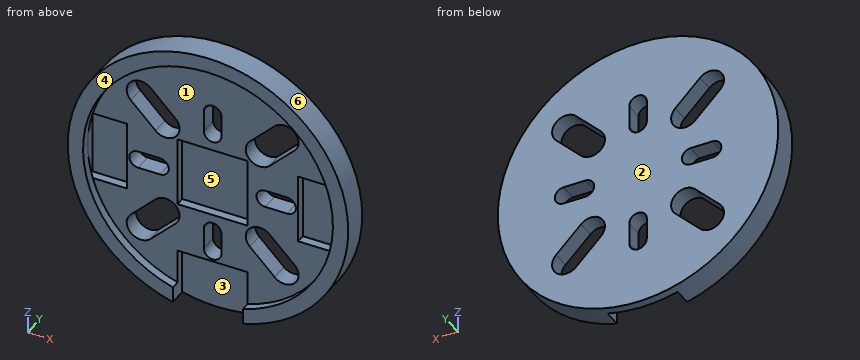
from build123d import *

# Parameters (mm, degrees)
F0_R     = 16
F1_DEPTH = 3
F3_DEPTH = 1
F4_W     = 8
F4_H     = 8
F4_W_2   = 4.5
F5_DEPTH = 1
F7_DEPTH = 3.001
F9_DEPTH = 3.001


with BuildPart() as f1:
    # F0 (on Front) → F1 (new body)
    with BuildSketch(Plane.XZ):
        Circle(F0_R)
    extrude(amount=F1_DEPTH)

    # F2 (on face) → F3 (cut)
    with BuildSketch(Plane.XZ.offset(3)):
        with BuildLine():
            Line((4, -16.6770793666), (4, -13.6770793666))
            ThreePointArc((4, -13.6770793666), (0, 14.25), (-4, -13.6770793666))
            Line((-4, -13.6770793666), (-4, -16.6770793666))
            Line((-4, -16.6770793666), (4, -16.6770793666))
        make_face()
    extrude(amount=-F3_DEPTH, mode=Mode.SUBTRACT)

    # F4 (on face) → F5 (cut)
    with BuildSketch(Plane.XZ.offset(2)):
        Rectangle(F4_W, F4_H)
        with Locations((-12, 0)):
            Rectangle(F4_W_2, F4_H)
        with Locations((12, 0)):
            Rectangle(F4_W_2, F4_H)
        with BuildLine():
            Line((4, -13.6770793666), (4, -9.75))
            Line((4, -9.75), (-4, -9.75))
            Line((-4, -9.75), (-4, -13.6770793666))
            Line((-4, -13.6770793666), (-4, -14.25))
            Line((-4, -14.25), (-4, -15.4919333848))
            ThreePointArc((-4, -15.4919333848), (0, -16), (4, -15.4919333848))
            Line((4, -15.4919333848), (4, -14.25))
            Line((4, -14.25), (4, -13.6770793666))
        make_face()
    extrude(amount=-F5_DEPTH, mode=Mode.SUBTRACT)

    # F6 (on face) → F7 (cut, through all)
    with BuildSketch(Plane(origin=(0, 0, 0), x_dir=(-1, 0, 0), z_dir=(0, 1, 0))):
        with BuildLine():
            Line((1, 6), (1, 8.5))
            ThreePointArc((1, 8.5), (0, 9.5), (-1, 8.5))
            Line((-1, 8.5), (-1, 6))
            ThreePointArc((-1, 6), (0, 5), (1, 6))
        make_face()
        with BuildLine():
            ThreePointArc((-8.5, 1), (-9.5, 0), (-8.5, -1))
            Line((-8.5, -1), (-6, -1))
            ThreePointArc((-6, -1), (-5, 0), (-6, 1))
            Line((-6, 1), (-8.5, 1))
        make_face()
        with BuildLine():
            ThreePointArc((-1, -8.5), (0, -9.5), (1, -8.5))
            Line((1, -8.5), (1, -6))
            ThreePointArc((1, -6), (0, -5), (-1, -6))
            Line((-1, -6), (-1, -8.5))
        make_face()
        with BuildLine():
            ThreePointArc((8.5, -1), (9.5, 0), (8.5, 1))
            Line((8.5, 1), (6, 1))
            ThreePointArc((6, 1), (5, 0), (6, -1))
            Line((6, -1), (8.5, -1))
        make_face()
    extrude(amount=-F7_DEPTH, mode=Mode.SUBTRACT)

    # F8 (on face) → F9 (cut, through all)
    with BuildSketch(Plane(origin=(0, 0, 0), x_dir=(-1, 0, 0), z_dir=(0, 1, 0))):
        with BuildLine():
            ThreePointArc((-7.0710678119, -9.3338095117), (-6.7242314097, -8.8147321535), (-6.6024386618, -8.2024386618))
            ThreePointArc((-6.6024386618, -8.2024386618), (-7.59014517, -6.7242314097), (-9.3338095117, -7.0710678119))
            ThreePointArc((-9.3338095117, -7.0710678119), (-9.3338095117, -9.3338095117), (-7.0710678119, -9.3338095117))
        make_face()
        with BuildLine():
            ThreePointArc((-9.3338095117, -7.0710678119), (-7.59014517, -6.7242314097), (-6.6024386618, -8.2024386618))
            ThreePointArc((-6.6024386618, -8.2024386618), (-6.7242314097, -8.8147321535), (-7.0710678119, -9.3338095117))
            Line((-7.0710678119, -9.3338095117), (-4.2426406871, -6.5053823869))
            ThreePointArc((-4.2426406871, -6.5053823869), (-6.5053823869, -6.5053823869), (-6.5053823869, -4.2426406871))
            Line((-6.5053823869, -4.2426406871), (-9.3338095117, -7.0710678119))
        make_face()
        with BuildLine():
            ThreePointArc((-3.774011537, -5.374011537), (-4.7617180452, -3.895804285), (-6.5053823869, -4.2426406871))
            ThreePointArc((-6.5053823869, -4.2426406871), (-6.5053823869, -6.5053823869), (-4.2426406871, -6.5053823869))
            ThreePointArc((-4.2426406871, -6.5053823869), (-3.895804285, -5.9863050288), (-3.774011537, -5.374011537))
        make_face()
        with BuildLine():
            Line((9.3338095117, -7.0710678119), (6.5053823869, -4.2426406871))
            ThreePointArc((6.5053823869, -4.2426406871), (6.852218789, -4.7617180452), (6.974011537, -5.374011537))
            ThreePointArc((6.974011537, -5.374011537), (5.9863050288, -6.852218789), (4.2426406871, -6.5053823869))
            Line((4.2426406871, -6.5053823869), (7.0710678119, -9.3338095117))
            ThreePointArc((7.0710678119, -9.3338095117), (7.0710678119, -7.0710678119), (9.3338095117, -7.0710678119))
        make_face()
        with BuildLine():
            ThreePointArc((6.974011537, -5.374011537), (6.852218789, -4.7617180452), (6.5053823869, -4.2426406871))
            ThreePointArc((6.5053823869, -4.2426406871), (4.2426406871, -4.2426406871), (4.2426406871, -6.5053823869))
            ThreePointArc((4.2426406871, -6.5053823869), (5.9863050288, -6.852218789), (6.974011537, -5.374011537))
        make_face()
        with BuildLine():
            ThreePointArc((9.8024386618, -8.2024386618), (9.6806459138, -7.59014517), (9.3338095117, -7.0710678119))
            ThreePointArc((9.3338095117, -7.0710678119), (7.0710678119, -7.0710678119), (7.0710678119, -9.3338095117))
            ThreePointArc((7.0710678119, -9.3338095117), (8.8147321535, -9.6806459138), (9.8024386618, -8.2024386618))
        make_face()
        with BuildLine():
            Line((7.0710678119, 9.3338095117), (4.2426406871, 6.5053823869))
            ThreePointArc((4.2426406871, 6.5053823869), (5.9863050288, 6.852218789), (6.974011537, 5.374011537))
            ThreePointArc((6.974011537, 5.374011537), (6.852218789, 4.7617180452), (6.5053823869, 4.2426406871))
            Line((6.5053823869, 4.2426406871), (9.3338095117, 7.0710678119))
            ThreePointArc((9.3338095117, 7.0710678119), (7.0710678119, 7.0710678119), (7.0710678119, 9.3338095117))
        make_face()
        with BuildLine():
            ThreePointArc((6.974011537, 5.374011537), (5.9863050288, 6.852218789), (4.2426406871, 6.5053823869))
            ThreePointArc((4.2426406871, 6.5053823869), (4.2426406871, 4.2426406871), (6.5053823869, 4.2426406871))
            ThreePointArc((6.5053823869, 4.2426406871), (6.852218789, 4.7617180452), (6.974011537, 5.374011537))
        make_face()
        with BuildLine():
            ThreePointArc((9.8024386618, 8.2024386618), (8.8147321535, 9.6806459138), (7.0710678119, 9.3338095117))
            ThreePointArc((7.0710678119, 9.3338095117), (7.0710678119, 7.0710678119), (9.3338095117, 7.0710678119))
            ThreePointArc((9.3338095117, 7.0710678119), (9.6806459138, 7.59014517), (9.8024386618, 8.2024386618))
        make_face()
        with BuildLine():
            Line((-9.3338095117, 7.0710678119), (-6.5053823869, 4.2426406871))
            ThreePointArc((-6.5053823869, 4.2426406871), (-6.5053823869, 6.5053823869), (-4.2426406871, 6.5053823869))
            Line((-4.2426406871, 6.5053823869), (-7.0710678119, 9.3338095117))
            ThreePointArc((-7.0710678119, 9.3338095117), (-6.7242314097, 8.8147321535), (-6.6024386618, 8.2024386618))
            ThreePointArc((-6.6024386618, 8.2024386618), (-7.59014517, 6.7242314097), (-9.3338095117, 7.0710678119))
        make_face()
        with BuildLine():
            ThreePointArc((-4.2426406871, 6.5053823869), (-6.5053823869, 6.5053823869), (-6.5053823869, 4.2426406871))
            ThreePointArc((-6.5053823869, 4.2426406871), (-4.7617180452, 3.895804285), (-3.774011537, 5.374011537))
            ThreePointArc((-3.774011537, 5.374011537), (-3.895804285, 5.9863050288), (-4.2426406871, 6.5053823869))
        make_face()
        with BuildLine():
            ThreePointArc((-7.0710678119, 9.3338095117), (-9.3338095117, 9.3338095117), (-9.3338095117, 7.0710678119))
            ThreePointArc((-9.3338095117, 7.0710678119), (-7.59014517, 6.7242314097), (-6.6024386618, 8.2024386618))
            ThreePointArc((-6.6024386618, 8.2024386618), (-6.7242314097, 8.8147321535), (-7.0710678119, 9.3338095117))
        make_face()
    extrude(amount=-F9_DEPTH, mode=Mode.SUBTRACT)


solid = f1.part
Could you check a few things on this model? Use its own coordinates, in mm. Face numbers are marked on the shaded views. A direction names the side the tool comes from. Round coordinates to 2 decimals unless told otherwise and drop trailing zeros. Order: outer loops, then holes, each group sorted by start corner. A loop starts at its lowest first (then second) coordinate and runs counter-clockwise, first axis right, second up. Notation, with made-up numbers: M 69,43.5 L 95,43.5 A22 cw 95,72.5 Z; hole C 85,-2.75 d8. An arc over 180 degrees is marked long. One line per item, written item: value.
(1) If we mould it in two halves opening along Z, with no side actions, what happens to the marked faces 4, 5 and 6? For each: released by +Z, released by -Z, zero draft, split by the parting line, or undercut.
Ans:
face 4: zero draft
face 5: undercut
face 6: split by the parting line
(2) I need wall thicknesses on line 1 along X through (y, z) = (-2.2, 0); line 2 along Z through (x, y) = (6, -1.8); line 3 along X through (y, z) = (-1.4, -4.5). Which ranges of each line are inside material? Lowest first, please. Write a range as from..to.
Ans:
line 1: x = -16..-14.25, 14.25..16
line 2: z = -14.83..-8.26, -3.9..-1, 1..3.9, 8.26..14.83
line 3: x = -15.35..-6.76, -4.03..4.03, 6.76..15.35
(3) Imagine slicing it at C-C (y = -2.55). Write out the boundary of the cut face in (x, z).
Ans:
outline: M -4,-15.49 L -4,-13.68 A14.25 cw long 4,-13.68 L 4,-15.49 A16 ccw long Z
(4) Imagine slicing it at A-A (x = 0). Write out the boundary of the cut face in (y, z), and give its area (3 significant figures).
Ans:
outline: M -3,14.25 L -2,14.25 L -2,9.5 L 0,9.5 L 0,16 L -3,16 Z; M -2,-9.75 L -1,-9.75 L -1,-16 L 0,-16 L 0,-9.5 L -2,-9.5 Z; M -2,-5 L 0,-5 L 0,5 L -2,5 L -2,4 L -1,4 L -1,-4 L -2,-4 Z
area: 33.5 mm^2
(5) Imagine slicing it at D-D (x = -5.5). Write out the boundary of the cut face in (y, z).
Ans:
outline: M -3,-15.02 L 0,-15.02 L 0,-7.76 L -2,-7.76 L -2,-13.15 L -3,-13.15 Z; M -3,13.15 L -2,13.15 L -2,7.76 L 0,7.76 L 0,15.02 L -3,15.02 Z; M -2,-3.78 L 0,-3.78 L 0,-0.87 L -2,-0.87 Z; M -2,0.87 L 0,0.87 L 0,3.78 L -2,3.78 Z
(6) Which directions (+Z, -Z, +X, -X, +Y, -Y) give clear straight access to the entire face, cutting with the end or side of a thin tool? Please do the marked faces 1, 2 and 3.
Ans:
face 1: -Y
face 2: +Z, -Z, +X, -X, +Y
face 3: -Z, -Y
(7) Imagine slicing it at B-B (z = -7.5). Write out the boundary of the cut face in (x, y), and give its area (3 significant figures).
Ans:
outline: M -14.13,-3 L -12.12,-3 L -12.12,-2 L -9.64,-2 L -9.64,0 L -14.13,0 Z; M -5.24,-2 L -1,-2 L -1,0 L -5.24,0 Z; M 1,-2 L 5.24,-2 L 5.24,0 L 1,0 Z; M 9.64,-2 L 12.12,-2 L 12.12,-3 L 14.13,-3 L 14.13,0 L 9.64,0 Z
area: 39.0 mm^2
(8) I'm going to push flat-ended pins straight in: P1, Ø0.8, axis at x = 1.5, y = -1.5, coming from the +Z side; P2, Ø1.9, axis at x = 0, z = -12.5, coming from the -Y side; P3, Ø1.5, axis at y = -2.5, z = -3, coming from the +X side. Where does each tip first touch, or does it pass through?
Ans:
P1: stops at z = 15.96
P2: stops at y = -1
P3: stops at x = 15.84
